Part model, mm, in its own coordinate system. A direction names the side the tool comes from. Round coordinates to 2 decimals unless told otherwise and drop trailing zeros. Loops run counter-clockwise (first coordinate to the right, second up) from the corner with the lowest first, then second, coordinate; pieces in that order, holes last.
(1) Cut at C-C on z = -2. List the corners of the cut face in (x, y).
(2) Cut at A-A on z = 37. List the corners of the cut face in (x, y).
(3) Flat gauge pins, fed straight in: pin 1 (2 mm diameter, centred on y = -3.5, z = 30, fed in from +X); pin 2 (2 mm diameter, centred on x = -1, y = 1.5, fed in from +Z); pin 3 (1 mm diameter, centred on x = -1, z = 1, fed in from -Y). Where does each tip first touch, or does it go through?
(4) Probe probe 1 along Y at (x, z) = (0, 43.65); probe 2 along Y at (x, z) = (0, 35); probe 3 along X at (y, z) = (0.25, 16). List the from-to ranges inside material, lowest first.
(5) Mould opens along Z. For faces 4 (the face through (0, 0, -5.5)), 5 (the face through (-3.233, -1.341, 37.177)), 6 (the face through (3.233, 1.341, -0.254)) say: +Z half, -Z half, draft (parallel to the pull), parting line (faces both ways), or undercut.
(6) Cut at B-B on z = 25. List the corners of the cut face in (x, y).
(7) Tool access for faces 1 (the face through (0, -4, 0)), 2 (the face through (0.867, -3.905, -2.472)), 3 (the face through (2.285, 3.584, 43.76)): list every direction of +Z, -Z, +X, -X, +Y, -Y with a clear straight run to the whole face (end or side of a thin tool).
from build123d import *

# Parameters (mm, degrees)
SKETCH_1_R                = 5.4
EXTRUDE_1_DEPTH           = 45
EXTRUDE_3_DEPTH           = 5.4
M8X1_0_TAPPED_HOLE1_D     = 7
M8X1_0_TAPPED_HOLE1_DEPTH = 13
M8X1_0_TAPPED_HOLE1_TIP   = 2.103012167
M3_TAPPED_HOLE1_D         = 2.5
M3_TAPPED_HOLE1_DEPTH     = 7.5
M3_TAPPED_HOLE1_TIP       = 0.751075774
CHAMFER_1_SIZE            = 0.5
CHAMFER_2_SIZE            = 0.5
SKETCH_9_R                = 4.25
CUT_EXTRUDE_5_DEPTH       = 2
CHAMFER_3_SIZE            = 0.5
SKETCH_10_W               = 90.830281396
SKETCH_10_H               = 34.560289278
CUT_EXTRUDE_1_DEPTH       = 85
EXTRUDE_START             = 0.5
SKETCH_11_R               = 3.5
EXTRUDE_1_2_DEPTH         = 0.5
SKETCH_12_R               = 4
EXTRUDE_2_DEPTH           = 5
CHAMFER_4_SIZE            = 1


with BuildPart() as part:
    # 草图1 → Extrude 1 (new body)
    with BuildSketch(Plane.XY):
        with Locations(Location((0, 0, 0), (0, 0, 180))):
            Circle(SKETCH_1_R)
    extrude(amount=EXTRUDE_1_DEPTH)

    # 草图4 → 拉伸3 (add, symmetric)
    with BuildSketch(Plane.XZ):
        with BuildLine():
            Line((-22, 0), (22, 0))
            Line((22, 0), (28, -15.05119142))
            ThreePointArc((28, -15.05119142), (0, -12), (-28, -15.05119142))
            Line((-28, -15.05119142), (-22, 0))
        make_face()
    extrude(amount=EXTRUDE_3_DEPTH, both=True)

    # M8x1.0 Tapped Hole1
    with Locations(Plane.XY.offset(45)):
        with Locations((0, 0)):
            Hole(M8X1_0_TAPPED_HOLE1_D / 2, depth=M8X1_0_TAPPED_HOLE1_DEPTH)
            with Locations((0, 0, -(M8X1_0_TAPPED_HOLE1_DEPTH + M8X1_0_TAPPED_HOLE1_TIP / 2))):  # 118° drill point
                Cone(0, M8X1_0_TAPPED_HOLE1_D / 2, M8X1_0_TAPPED_HOLE1_TIP, mode=Mode.SUBTRACT)

    # M3 Tapped Hole1
    with Locations(Plane(origin=(-19.5, -1.4, 0), x_dir=(0, 1, 0), z_dir=(0, 0, 1))):
        with Locations((0, 0), (0, -39)):
            Hole(M3_TAPPED_HOLE1_D / 2, depth=M3_TAPPED_HOLE1_DEPTH)
            with Locations((0, 0, -(M3_TAPPED_HOLE1_DEPTH + M3_TAPPED_HOLE1_TIP / 2))):  # 118° drill point
                Cone(0, M3_TAPPED_HOLE1_D / 2, M3_TAPPED_HOLE1_TIP, mode=Mode.SUBTRACT)

    # 倒角1
    chamfer_1_edges = [part.edges().sort_by_distance(p)[0] for p in [
        (19.5, -0.15, 0),
        (-19.5, -0.15, 0),
    ]]
    chamfer(chamfer_1_edges, length=CHAMFER_1_SIZE)

    # 倒角2
    chamfer_2_edges = [part.edges().sort_by_distance(p)[0] for p in [
        (5.4, 0, 45),
    ]]
    chamfer(chamfer_2_edges, length=CHAMFER_2_SIZE)

    # 草图9 → 拉伸5 (cut)
    with BuildSketch(Plane.XY.offset(45)):
        Circle(SKETCH_9_R)
    extrude(amount=-CUT_EXTRUDE_5_DEPTH, mode=Mode.SUBTRACT)

    # 倒角3
    chamfer_3_edges = [part.edges().sort_by_distance(p)[0] for p in [
        (-4.25, 0, 45),
        (3.5, 0, 43),
    ]]
    chamfer(chamfer_3_edges, length=CHAMFER_3_SIZE)

    # 草图10 → 切除-拉伸1 (cut)
    with BuildSketch(Plane.XY):
        Rectangle(SKETCH_10_W, SKETCH_10_H)
    extrude(amount=-CUT_EXTRUDE_1_DEPTH, mode=Mode.SUBTRACT)

    # 草图11 → Extrude 1 2 (add)
    with BuildSketch(Plane(origin=(0, 0, 0), x_dir=(-1, 0, 0), z_dir=(0, 0, -1)).offset(EXTRUDE_START)):
        with Locations(Location((0, 0, 0), (0, 0, 180))):
            Circle(SKETCH_11_R)
    extrude(amount=-EXTRUDE_1_2_DEPTH)

    # 草图12 → 凸台-拉伸2 (add)
    with BuildSketch(Plane(origin=(0, 0, -0.5), x_dir=(-1, 0, 0), z_dir=(0, 0, -1))):
        Circle(SKETCH_12_R)
    extrude(amount=EXTRUDE_2_DEPTH)

    # 倒角4
    chamfer_4_edges = [part.edges().sort_by_distance(p)[0] for p in [
        (4, 0, -5.5),
    ]]
    chamfer(chamfer_4_edges, length=CHAMFER_4_SIZE)


solid = part.part
Final values:
1. outline: circle Ø8 at (0, 0)
2. outline: circle Ø10.8 at (0, 0); hole circle Ø7 at (0, 0)
3. pin 1: stops at x = 4.79
3. pin 2: stops at z = 31.58
3. pin 3: stops at y = -5.38
4. probe 1: y = -5.4 to -4.25, 4.25 to 5.4
4. probe 2: y = -5.4 to -3.5, 3.5 to 5.4
4. probe 3: x = -5.39 to 5.39
5. face 4: -Z half
5. face 5: draft
5. face 6: undercut
6. outline: circle Ø10.8 at (0, 0)
7. face 1: none
7. face 2: -Z
7. face 3: +Z
